Work out the finished part from the listing and answer in its coordinate system (mm). Face numbers are marked on the shaded views. Give positions to 0.01 mm unless a question says otherwise; leave off trailing zeros. Write each loop counter-clockwise with the first axis right and the second up, starting at its lowest first coordinate (ties: lowest second). Pieces come first, ordered by that corner, then holes.
1) Determine the mould class of the marked faces 1, 2 and 3 for opening direction Z: pulls with the +Z half, pulls with the -Z half, needs draft (parallel to the pull), parting line crosses it, or undercut.
2) Find section C-C (y = 1.75). Determine the outline of the cut face in (x, z), plus the area to 3 significant figures.
3) Find section B-B (z = 0). Determine the outline of the cut face in (x, y), plus the area to 3 significant figures.
4) Straight lines are drawn through the part: probe 1 along X at (y, z) = (-3.2, 0); probe 2 along X at (y, z) = (2.95, 0); probe 3 along Z at (x, y) = (-9.5, -0.5). For each, find the intervals that lie inside material, in ascending order.
5) Given pin 1 Ø4 at (x, y) = (7, 3.5) entering from +Z; pin 2 Ø1.5 at (y, z) = (0.5, 12) entering from -X; pin 3 Ø2 at (y, z) = (-0.5, -11) entering from -X, each flat-ended and moving along its own axis, determine where each tip first touches the part or whether it passes through.
6) Find section A-A (x = 0). Determine the outline of the cut face in (y, z).
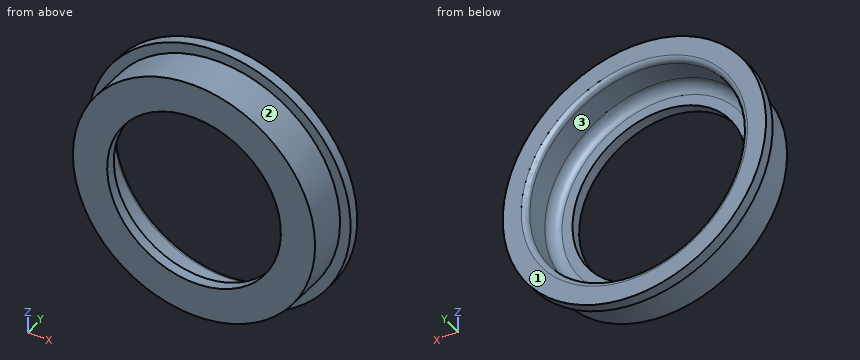
```python
from build123d import *


with BuildPart() as part:
    # Esquisse1 → Révolution1 (revolve)
    with BuildSketch(Plane.XY, mode=Mode.PRIVATE) as r_volution1_sk:
        with BuildLine():
            Line((-16.5, -4), (-16.5, -2))
            Line((-16.5, -2), (-18.5, -2))
            ThreePointArc((-18.5, -2), (-19.914213562, -1.414213562), (-20.5, 0))
            Line((-20.5, 0), (-20.5, 4.5))
            ThreePointArc((-20.5, 4.5), (-20.792893219, 5.207106781), (-21.5, 5.5))
            Line((-21.5, 5.5), (-25, 5.5))
            Line((-25, 5.5), (-25, 3.5))
            Line((-25, 3.5), (-23, 3.5))
            Line((-23, 3.5), (-23, -4))
            Line((-23, -4), (-16.5, -4))
        make_face()
    revolve(r_volution1_sk.sketch.rotate(Axis((0, 27.606261023, 0), (0, -1, 0)), 270), axis=Axis((0, 27.606261023, 0), (0, -1, 0)))  # turned: the seam where the file's is


solid = part.part
```
Results:
1. face 1: needs draft
1. face 2: parting line crosses it
1. face 3: undercut
2. outline: circle Ø46 at (0, 0); hole circle Ø41 at (0, 0)
2. area: 342 mm2
3. outline: (-25, 3.5) - (-23, 3.5) - (-23, -4) - (-16.5, -4) - (-16.5, -2) - (-18.5, -2) arc R2 cw to (-20.5, 0) - (-20.5, 4.5) arc R1 ccw to (-21.5, 5.5) - (-25, 5.5) - close; (16.5, -4) - (23, -4) - (23, 3.5) - (25, 3.5) - (25, 5.5) - (21.5, 5.5) arc R1 ccw to (20.5, 4.5) - (20.5, 0) arc R2 cw to (18.5, -2) - (16.5, -2) - close
3. area: 72.8 mm2
4. probe 1: x = -23 to -16.5, 16.5 to 23
4. probe 2: x = -23 to -20.5, 20.5 to 23
4. probe 3: z = -20.95 to -18.09, 18.09 to 20.95
5. pin 1: stops at z = 24.49
5. pin 2: stops at x = -20.06
5. pin 3: stops at x = -20.71
6. outline: (-4, -23) - (3.5, -23) - (3.5, -25) - (5.5, -25) - (5.5, -21.5) arc R1 ccw to (4.5, -20.5) - (0, -20.5) arc R2 cw to (-2, -18.5) - (-2, -16.5) - (-4, -16.5) - close; (-4, 16.5) - (-2, 16.5) - (-2, 18.5) arc R2 cw to (0, 20.5) - (4.5, 20.5) arc R1 ccw to (5.5, 21.5) - (5.5, 25) - (3.5, 25) - (3.5, 23) - (-4, 23) - close
